Geometry: see drawing. Coordinates: mm, zero at the bounding-box minimum. A direction names the side the tool comes from. Round coordinates to 2 decimals unless told otherwise and drop trailing zeros. Loops run counter-clockwise (first coordinate to the right, second up) from the corner with the lowest first, then second, coordinate; pieces in that order, holes last.
(1) Section B-B, the plane y = 4. Return the cut outline in (x, z), plus the area to 3 significant figures.
(2) Set-up query: the marked faces 1 and 2. Return all of +Z, -Z, +X, -X, +Y, -Y with unobstructed straight access to the full face (end or side cutting, diameter ignored); none if empty.
(3) Material intervals for probe 1 along X at (y, z) = (3.25, 4); probe 2 along Y at (x, z) = (11, 3.25), sorted ascending.
(4) Section C-C, the plane x = 6. Return the cut outline in (y, z).
(5) Section A-A, the plane z = 4. Return the cut outline in (x, y).
(6) Mould query, pull axis Z, two halves, no side actions, for the marked faces 3, 4 and 5. Classes: pulls with the +Z half, pulls with the -Z half, needs draft (parallel to the pull), parting line crosses it, or undercut.
(7) Section D-D, the plane x = 3.75. Return the cut outline in (y, z).
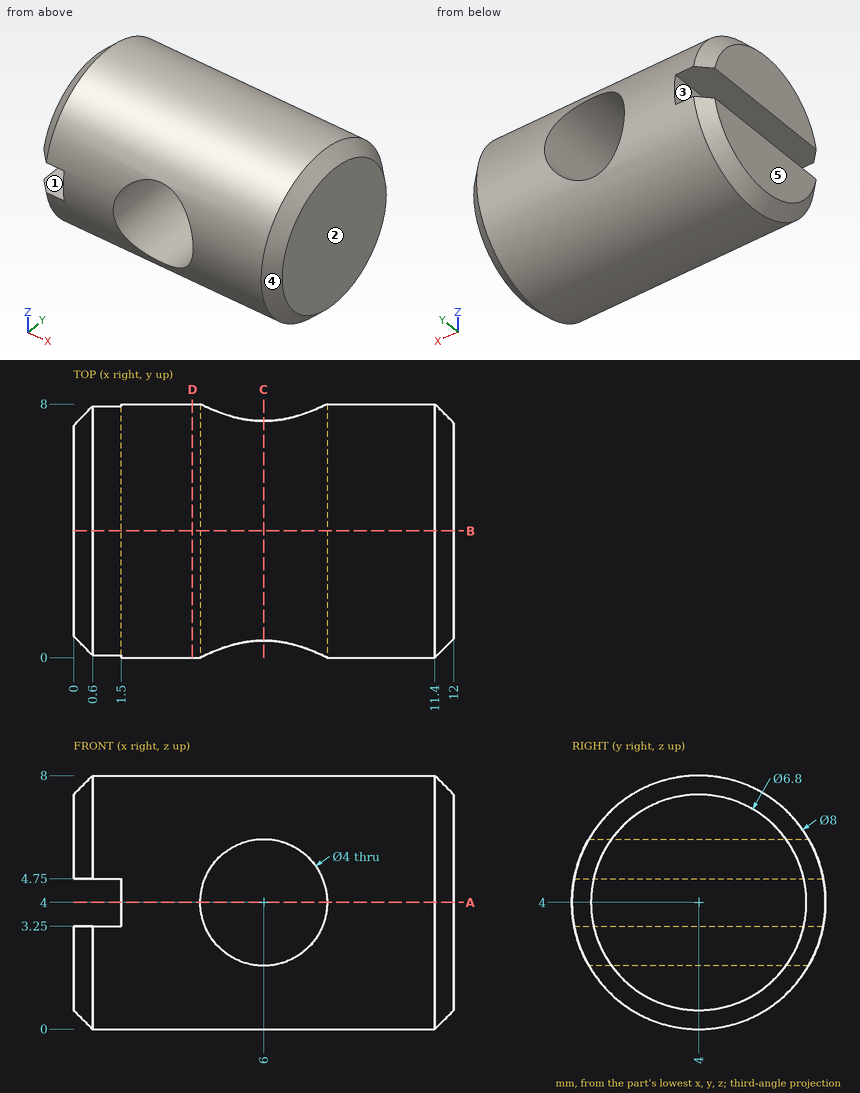
Output values:
1. outline: (0, 0.6) - (0.6, 0) - (11.4, 0) - (12, 0.6) - (12, 7.4) - (11.4, 8) - (0.6, 8) - (0, 7.4) - (0, 4.75) - (1.5, 4.75) - (1.5, 3.25) - (0, 3.25) - close; hole circle Ø4 at (6, 4)
1. area: 80.5 mm2
2. face 1: -X, +Y, -Y
2. face 2: +Z, -Z, +X, +Y, -Y
3. probe 1: x = 1.5 to 4, 8 to 12
3. probe 2: y = 0.07 to 7.93
4. outline: (0.54, 2) arc R4 ccw to (7.46, 2) - close; (0.54, 6) - (7.46, 6) arc R4 ccw to start
5. outline: (1.5, 0) - (4, 0) - (4, 8) - (1.5, 8) - close; (8, 0) - (11.4, 0) - (12, 0.6) - (12, 7.4) - (11.4, 8) - (8, 8) - close
6. face 3: undercut
6. face 4: parting line crosses it
6. face 5: needs draft
7. outline: circle Ø8 at (4, 4)
